from build123d import *

# Parameters (mm, degrees)
BOSS_EXTRUDE1_DEPTH                      = 30
CUT_EXTRUDE1_DEPTH                       = 306.614135799
CUT_EXTRUDE1_DEPTH_BACK                  = 306.614135799
SKETCH2_R                                = 5
BOSS_EXTRUDE2_START                      = -10
BOSS_EXTRUDE2_DEPTH                      = 15
CBORE_FOR_M10_HEX_HEAD_BOLT1_D           = 10
CBORE_FOR_M10_HEX_HEAD_BOLT1_CBORE_D     = 15
CBORE_FOR_M10_HEX_HEAD_BOLT1_CBORE_DEPTH = 8


with BuildPart() as part:
    # Sketch1 → Boss-Extrude1 (new, symmetric)
    with BuildSketch(Plane(origin=(0, 0, 0), x_dir=(0, 0, -1), z_dir=(1, 0, 0))):
        with BuildLine():
            Line((0, 0), (0, 15))
            Line((0, 15), (47.251760651, 15))
            ThreePointArc((47.251760651, 15), (58.870710689, 19.252272915), (65, 30))
            Line((65, 30), (194.009804864, 30))
            ThreePointArc((194.009804864, 30), (221.395932739, 35.178799781), (245, 50))
            Line((245, 50), (280, 50))
            Line((280, 50), (300, 30))
            Line((300, 30), (300, -10))
            Line((300, -10), (245, -10))
            ThreePointArc((245, -10), (190.685134604, -2.505230148), (135.912878854, 0))
            Line((135.912878854, 0), (0, 0))
        make_face()
        Polygon((63, 7.5), (78, 22.5), (93, 7.5), align=None, mode=Mode.SUBTRACT)
        Polygon((104, 7.5), (89, 22.5), (119, 22.5), align=None, mode=Mode.SUBTRACT)
        Polygon((171, 22.5), (156, 7.5), (141, 22.5), align=None, mode=Mode.SUBTRACT)
        Polygon((145, 7.5), (115, 7.5), (130, 22.5), align=None, mode=Mode.SUBTRACT)
        Polygon((223, 22.5), (208, 7.5), (193, 22.5), align=None, mode=Mode.SUBTRACT)
        Polygon((197, 7.5), (167, 7.5), (182, 22.5), align=None, mode=Mode.SUBTRACT)
    extrude(amount=BOSS_EXTRUDE1_DEPTH, both=True)

    # Sketch2 → Cut-Extrude1 (cut, two sides: drawn at the far end of the back side and taken through both)
    with BuildSketch(Plane(origin=(0, 0, 0), x_dir=(1, 0, 0), z_dir=(0, 1, 0)).offset(-CUT_EXTRUDE1_DEPTH_BACK)):
        with BuildLine():
            ThreePointArc((15, 194), (15.855513863, 207.052619222), (18.407417371, 219.88190451))
            Line((18.407417371, 219.88190451), (30, 263.146011872))
            Line((30, 263.146011872), (30, 300))
            Line((30, 300), (100, 300))
            Line((100, 300), (100, 0))
            Line((100, 0), (0, 0))
            ThreePointArc((0, 0), (10.606601718, 4.393398282), (15, 15))
            Line((15, 15), (15, 194))
        make_face()
        with BuildLine():
            Line((-15, 15), (-15, 194))
            ThreePointArc((-15, 194), (-15.855513863, 207.052619222), (-18.407417371, 219.88190451))
            Line((-18.407417371, 219.88190451), (-30, 263.146011872))
            Line((-30, 263.146011872), (-30, 300))
            Line((-30, 300), (-100, 300))
            Line((-100, 300), (-100, 0))
            Line((-100, 0), (0, 0))
            ThreePointArc((0, 0), (-10.606601718, 4.393398282), (-15, 15))
        make_face()
        with BuildLine():
            Line((-20, 300), (20, 300))
            Line((20, 300), (20, 270))
            ThreePointArc((20, 270), (15.606601718, 259.393398282), (5, 255))
            Line((5, 255), (0, 255))
            Line((0, 255), (-5, 255))
            ThreePointArc((-5, 255), (-15.606601718, 259.393398282), (-20, 270))
            Line((-20, 270), (-20, 300))
        make_face()
        with Locations(Location((0, 15, 0), (0, 0, 270))):
            Circle(SKETCH2_R)
    extrude(amount=CUT_EXTRUDE1_DEPTH + CUT_EXTRUDE1_DEPTH_BACK, mode=Mode.SUBTRACT)

    # Sketch3 → Boss-Extrude2 (add)
    with BuildSketch(Plane(origin=(0, 0, 0), x_dir=(1, 0, 0), z_dir=(0, 1, 0)).offset(BOSS_EXTRUDE2_START)):
        with BuildLine():
            Line((-20, 270), (-20, 280))
            Line((-20, 280), (-20, 300))
            Line((-20, 300), (-30, 300))
            Line((-30, 300), (-35.78511038, 309.938938469))
            ThreePointArc((-35.78511038, 309.938938469), (-35.838126061, 329.969422485), (-18.5, 340))
            Line((-18.5, 340), (0, 340))
            Line((0, 340), (18.5, 340))
            ThreePointArc((18.5, 340), (35.838126061, 329.969422485), (35.78511038, 309.938938469))
            Line((35.78511038, 309.938938469), (30, 300))
            Line((30, 300), (20, 300))
            Line((20, 300), (20, 280))
            Line((20, 280), (20, 270))
            ThreePointArc((20, 270), (15.606601718, 259.393398282), (5, 255))
            Line((5, 255), (-5, 255))
            ThreePointArc((-5, 255), (-15.606601718, 259.393398282), (-20, 270))
        make_face()
    extrude(amount=BOSS_EXTRUDE2_DEPTH)

    # CBORE for M10 Hex Head Bolt1 (through all)
    with Locations(Plane(origin=(0, 5, 0), x_dir=(1, 0, 0), z_dir=(0, 1, 0))):
        with Locations((0, 280), (-18.45, 320), (18.45, 320)):
            CounterBoreHole(CBORE_FOR_M10_HEX_HEAD_BOLT1_D / 2, CBORE_FOR_M10_HEX_HEAD_BOLT1_CBORE_D / 2, CBORE_FOR_M10_HEX_HEAD_BOLT1_CBORE_DEPTH)


solid = part.part
Could you check a few things on this model? Use its own coordinates, in mm. A direction names the side the tool comes from. Give positions to 0.01 mm unless a question says otherwise; leave off trailing zeros. Order: outer loops, then holes, each group sorted by start corner. A loop starts at its lowest first (then second) coordinate and runs counter-clockwise, first axis right, second up.
1. Suppose I cut it at A-A (z = -320). Write out the boundary of the cut face in (x, y).
Answers below:
outline: (-38.5, -10) - (-23.45, -10) - (-23.45, -3) - (-25.95, -3) - (-25.95, 5) - (-38.5, 5) - close; (-13.45, -10) - (13.45, -10) - (13.45, -3) - (10.95, -3) - (10.95, 5) - (-10.95, 5) - (-10.95, -3) - (-13.45, -3) - close; (23.45, -10) - (38.5, -10) - (38.5, 5) - (25.95, 5) - (25.95, -3) - (23.45, -3) - close
2. Suppose I cut it at B-B (z = -81). Write out the boundary of the cut face in (x, y), plus the area to 3 significant figures.
Answers below:
outline: (-15, 0) - (15, 0) - (15, 7.5) - (-15, 7.5) - close; (-15, 19.5) - (15, 19.5) - (15, 30) - (-15, 30) - close
area: 540 mm2
3. I need wall thicknesses on L1, parallel to X at y = 1.75, z = -320; L2, parallel to X at y = -4.5, z = -320; L3, parallel to X at y = -5.75, z = -280. Which ranges of each line are inside material? Lowest first, please.
Answers below:
L1: x = -38.5 to -25.95, -10.95 to 10.95, 25.95 to 38.5
L2: x = -38.5 to -23.45, -13.45 to 13.45, 23.45 to 38.5
L3: x = -30 to -5, 5 to 30
4. For pin 1 (1 mm diameter, centred on x = -16, y = 43, fed in from -Z); pin 2 (15 mm diameter, centred on x = 0, z = -183, fed in from +Y); pin 3 (1.5 mm diameter, centred on y = 14.5, z = -265, fed in from +X); pin 4 (6 mm diameter, centred on y = -4, z = -43.5, fed in from +X), each with a flat end and sliding along its axis, tell me the tip position at first contact or that it passes through.
Answers below:
pin 1: stops at z = -260.37
pin 2: stops at y = 30
pin 3: stops at x = 30
pin 4: passes through
5. Thinking about a two-plate mould opening in Y: for faces 1 (the flat face through (0, 27, -255)), 2 (the flat face through (-25, 40, -290)), 3 (the flat face through (0, 22.5, -156)), which applies, +Y half, -Y half, draft (parallel to the pull), parting line (faces both ways), or undercut?
Answers below:
face 1: draft
face 2: +Y half
face 3: undercut
6. Suppose I cut it at D-D (z = -36). Write out the boundary of the cut face in (x, y), plus the area to 3 significant figures.
Answers below:
outline: (-15, 0) - (15, 0) - (15, 15) - (-15, 15) - close
area: 450 mm2
7. Suppose I cut it at C-C (y = 41.5). Write out the boundary of the cut face in (x, z), plus the area to 3 significant figures.
Answers below:
outline: (-30, -288.5) - (-20, -288.5) - (-20, -270) arc R15 cw to (-5, -255) - (5, -255) arc R15 cw to (20, -270) - (20, -288.5) - (30, -288.5) - (30, -263.15) - (22.17, -233.92) - (-22.17, -233.92) - (-30, -263.15) - close
area: 1,800 mm2
8. Which directions (+Z, -Z, +X, -X, +Y, -Y) give clear straight access to the entire face, cutting with the end or side of a thin tool? Please do faces 4 (the cylindrical face through (16.82, 1.06, -312.68)), 5 (the flat face through (15, 6, -103)), 6 (the flat face through (-20, 22, -285)), 7 (the flat face through (-15, 6, -103)), 8 (the flat face through (0, 0, -69)).
Answers below:
face 4: +Y
face 5: +Z, +X, +Y, -Y
face 6: -Z, +Y
face 7: +Z, -X, +Y, -Y
face 8: +Z, +X, -X, -Y
